Source: CAD feature listing. Evaluate the final solid. Frame: model axes, mm. A direction names the side the tool comes from. Coordinates: 2 decimals unless noted, no trailing zeros. Write each loop counter-clockwise with the first axis right and the second up, starting at its lowest first coordinate (ties: lowest second). Pieces come first, ordered by that corner, then holes. Notation, with made-up numbers: (57.25, 78.25) -> (100.25, 78.25) arc R15 cw to (100.25, 104.25) -> close; hole circle Ø9 at (52, 58.25). An arc over 180 degrees is marked (long way). Write item = value, one per line.
from build123d import *

# Parameters (mm, degrees)
PAD009_DEPTH          = 23
PAD010_DEPTH          = 44
SKETCH024_W           = 43
SKETCH024_H           = 50
POCKET012_DEPTH       = 46
PAD011_DEPTH          = 25
SKETCH026_R           = 1.5
POCKET013_DEPTH       = 44.001
SKETCH027_R           = 3
POCKET014_DEPTH       = 10
POLARPATTERN001_COUNT = 4
POCKET011_DEPTH       = 6
PAD008_DEPTH          = 44
POCKET015_DEPTH       = 64.001
PAD013_DEPTH          = 64
SKETCH032_W           = 40
SKETCH032_H           = 10.43081
POCKET016_DEPTH       = 23.545613
SKETCH033_R           = 1.5
POCKET017_DEPTH       = 83.001
SKETCH034_R           = 4
POCKET018_DEPTH       = 80.001
SKETCH036_R           = 1.5
POCKET019_DEPTH       = 5
SKETCH037_R           = 3
POCKET020_DEPTH       = 10
SKETCH052_W           = 20
SKETCH052_H           = 20
PAD024_DEPTH          = 5
FILLET_R              = 8
FILLET001_R           = 3


with BuildPart() as part:
    # Sketch022 → Pad009 (new body)
    with BuildSketch(Plane.XY):
        Polygon((32, -51), (32, 32), (-32, 32), (-32, -51), (-20, -51), (-20, 20), (20, 20), (20, -51), align=None)
    extrude(amount=-PAD009_DEPTH)

    # Sketch023 (on Face10 of Pad009) → Pad010 (join)
    with BuildSketch(Plane(origin=(0, 0, -23), x_dir=(1, 0, 0), z_dir=(0, 0, -1))):
        with BuildLine():
            Line((-25, 51), (-25, -1))
            Line((-25, -1), (25, -1))
            Line((25, -1), (25, 51))
            Line((25, 51), (11.999997, 51))
            Line((11.999997, 27.99216), (11.999997, 51))
            ThreePointArc((-11.999997, 28.007844), (-0.007842, 16.000003), (11.999997, 27.99216))
            Line((-11.999997, 28.007844), (-11.999997, 51))
            Line((-11.999997, 51), (-25, 51))
        make_face()
    extrude(amount=PAD010_DEPTH)

    # Sketch024 (on Face18 of Pad010) → Pocket012 (cut)
    with BuildSketch(Plane.XZ.offset(51)):
        with Locations((-0.015156, -53)):
            Rectangle(SKETCH024_W, SKETCH024_H)
    extrude(amount=-POCKET012_DEPTH, mode=Mode.SUBTRACT)

    # Sketch025 (on Face14 of Pocket012) → Pad011 (join)
    with BuildSketch(Plane.XZ.offset(51)):
        Polygon((-32, -23), (-25, -23), (-25, -42.561909), align=None)
        Polygon((32, -23), (25, -23), (25, -42.561909), align=None)
    extrude(amount=-PAD011_DEPTH)

    # Sketch026 (on Face11 of Pad011) → Pocket013 (cut, through all)
    with BuildSketch(Plane.XY.offset(-23)):
        with Locations((-15.5, -12.5)):
            Circle(SKETCH026_R)
        with Locations((-15.5, -43.5)):
            Circle(SKETCH026_R)
        with Locations((15.5, -43.5)):
            Circle(SKETCH026_R)
        with Locations((15.5, -12.5)):
            Circle(SKETCH026_R)
    extrude(amount=-POCKET013_DEPTH, mode=Mode.SUBTRACT)

    # Sketch027 (on Face4 of Pocket013) → Pocket014 (cut)
    with BuildSketch(Plane.XY):
        with Locations((-25, 25)):
            Circle(SKETCH027_R)
    pocket014 = extrude(amount=-POCKET014_DEPTH, mode=Mode.SUBTRACT)

    # PolarPattern001: Pocket014 ×4 about axis
    polarpattern001_axis = Axis((0, 0, 0), (0, 0, 1))
    for i in range(1, POLARPATTERN001_COUNT):
        add(pocket014.rotate(polarpattern001_axis, i * 360 / POLARPATTERN001_COUNT), mode=Mode.SUBTRACT)

    # Sketch028 (on Face23 of PolarPattern001) → Pocket011 (cut)
    with BuildSketch(Plane(origin=(0, 1, 0), x_dir=(-1, 0, 0), z_dir=(0, 1, 0))):
        with BuildLine():
            Line((-11.999999, -62.717157), (12.000001, -62.717157))
            Line((12.000001, -62.717157), (12.000001, -49.356773))
            ThreePointArc((12.000001, -49.356773), (1e-06, -37.356773), (-11.999999, -49.356773))
            Line((-11.999999, -49.356773), (-11.999999, -62.717157))
        make_face()
    extrude(amount=-POCKET011_DEPTH, mode=Mode.SUBTRACT)

    # Sketch021 (on Face6 of Pocket011) → Pad008 (join)
    with BuildSketch(Plane(origin=(0, 0, -23), x_dir=(1, 0, 0), z_dir=(0, 0, -1))):
        Polygon((-32, 17), (-25, 17), (-25, 7), (-17, -1), (-17, -15), (-12, -20), (12, -20), (17, -15), (17, -1), (25, 7), (25, 17), (32, 17), (32, -27), (27, -32), (-27, -32), (-32, -27), align=None)
    extrude(amount=PAD008_DEPTH)

    # Sketch029 (on Face52 of Pad008) → Pocket015 (cut, through all)
    with BuildSketch(Plane(origin=(-32, 0, 0), x_dir=(0, -1, 0), z_dir=(-1, 0, 0))):
        with BuildLine():
            Line((7, 0), (-13, 0))
            Line((-13, -62), (-13, 0))
            Line((-13, -62), (0, -62))
            ThreePointArc((0, -62), (4.949747, -59.949747), (7, -55))
            Line((7, -55), (7, 0))
        make_face()
    extrude(amount=-POCKET015_DEPTH, mode=Mode.SUBTRACT)

    # Sketch031 (on Face10 of Pocket015) → Pad013 (join)
    with BuildSketch(Plane(origin=(-32, 0, 0), x_dir=(0, -1, 0), z_dir=(-1, 0, 0))):
        Polygon((51, 0), (51, 23.544613), (32.56919, 0), align=None)
    extrude(amount=-PAD013_DEPTH)

    # Sketch032 (on Face54 of Pad013) → Pocket016 (cut, through all)
    with BuildSketch(Plane(origin=(0, 0, 0), x_dir=(1, 0, 0), z_dir=(0, 0, -1))):
        with Locations((0, 37.784595)):
            Rectangle(SKETCH032_W, SKETCH032_H)
    extrude(amount=-POCKET016_DEPTH, mode=Mode.SUBTRACT)

    # Sketch033 (on Face19 of Pocket016) → Pocket017 (cut, through all)
    with BuildSketch(Plane.XZ.offset(51)):
        with Locations((-24.5, 8)):
            Circle(SKETCH033_R)
        with Locations((24.5, 8)):
            Circle(SKETCH033_R)
    extrude(amount=-POCKET017_DEPTH, mode=Mode.SUBTRACT)

    # Sketch034 (on Face19 of Pocket017) → Pocket018 (cut, through all)
    with BuildSketch(Plane.XZ.offset(48)):
        with Locations((-24.5, 8)):
            Circle(SKETCH034_R)
        with Locations((24.5, 8)):
            Circle(SKETCH034_R)
    extrude(amount=-POCKET018_DEPTH, mode=Mode.SUBTRACT)

    # Sketch036 (on Face6 of Pocket018) → Pocket019 (cut)
    with BuildSketch(Plane.XY.offset(-62)):
        with Locations((24.5, 7)):
            Circle(SKETCH036_R)
        with Locations((-24.5, 7)):
            Circle(SKETCH036_R)
    extrude(amount=-POCKET019_DEPTH, mode=Mode.SUBTRACT)

    # Sketch037 (on Face43 of Pocket019) → Pocket020 (cut)
    with BuildSketch(Plane.XY):
        with Locations((-24.5, 7)):
            Circle(SKETCH037_R)
        with Locations((24.5, 7)):
            Circle(SKETCH037_R)
    extrude(amount=-POCKET020_DEPTH, mode=Mode.SUBTRACT)

    # Sketch052 (on Face17 of Pocket020) → Pad024 (join)
    with BuildSketch(Plane.YZ.offset(32)):
        with Locations((3, -30)):
            Rectangle(SKETCH052_W, SKETCH052_H)
    pad024 = extrude(amount=-PAD024_DEPTH)

    # Mirrored002: Pad024 across YZ
    add(pad024.mirror(Plane.YZ))

    # Fillet
    fillet_edges = [part.edges().sort_by_distance(p)[0] for p in [
        (29.5, -7, -20),
        (29.5, 13, -20),
        (29.5, 13, -40),
        (29.5, -7, -40),
        (-29.5, -7, -20),
        (-29.5, 13, -20),
        (-29.5, -7, -40),
        (-29.5, 13, -40),
    ]]
    fillet(fillet_edges, radius=FILLET_R)

    # Fillet001
    fillet001_edges = [part.edges().sort_by_distance(p)[0] for p in [
        (24.5, 13, -62),
        (-24.5, 13, -62),
    ]]
    fillet(fillet001_edges, radius=FILLET001_R)


solid = part.part
1) Cut plane B-B, the plane z = -52. Output: boundary loops of the cut face in (x, y), and give its area (3 significant figures).
Answer block:
outline = (-32, -17) -> (-25, -17) -> (-25, -51) -> (-21.52, -51) -> (-21.52, -7) -> (-32, -7) -> close; (-32, 13) -> (-17, 13) -> (-17, 15) -> (-12, 20) -> (12, 20) -> (17, 15) -> (17, 13) -> (32, 13) -> (32, 27) -> (27, 32) -> (-27, 32) -> (-32, 27) -> close; (21.48, -51) -> (25, -51) -> (25, -17) -> (32, -17) -> (32, -7) -> (21.48, -7) -> close
area = 1,430 mm2
2) First-contact query: pin 1 Ø1 at (x, y) = (-11, -10) entering from +Z; pin 2 Ø10 at (y, z) = (-35.5, -35) entering from +X; pin 3 Ø6.5 at (x, y) = (-0.5, -46) entering from -Z. Flat tips, straight axial feed; report the tip coordinate or a pass-through.
Answer block:
pin_1 = -23
pin_2 = 29.5
pin_3 = 0
3) Cut plane C-C, the plane y = 25. Output: boundary loops of the cut face in (x, z), and give its area (3 significant figures).
Answer block:
outline = (-32, -67) -> (32, -67) -> (32, 0) -> (28, 0) -> (28, -10) -> (22, -10) -> (22, 0) -> (-22, 0) -> (-22, -10) -> (-28, -10) -> (-28, 0) -> (-32, 0) -> close
area = 4,170 mm2
4) Reachability of faces 4 (the flat face through (24, 5, -62)), 5 (the cylindrical face through (23.633, -43.303, 4.095)), 6 (the flat face through (28, -26, -30)), 7 (the flat face through (-12, -39, -25)), 8 (the cylindrical face through (15.175, -44.964, -25.465)) from +Z, -Z, +X, -X, +Y, -Y: full face, straight path, thin tool, end or side. Return the list, or none.
Answer block:
face_4 = +X, -X
face_5 = +Y
face_6 = -Z, +X
face_7 = -Z, -Y
face_8 = -Z
5) Cut plane A-A, the plane x = 15.5. Output: boundary loops of the cut face in (y, z), and give its area (3 significant figures).
Answer block:
outline = (-51, -28) -> (-45, -28) -> (-45, -23) -> (-51, -23) -> close; (-51, 0) -> (-43, 0) -> (-43, 13.32) -> (-51, 23.54) -> close; (-42, -28) -> (-14, -28) -> (-14, -23) -> (-42, -23) -> close; (-11, -28) -> (-7, -28) -> (-7, -23) -> (-11, -23) -> close; (-5, -67) -> (1, -67) -> (1, -62) -> (0, -62) arc R7 cw to (-5, -59.9) -> close; (16.5, -67) -> (32, -67) -> (32, 0) -> (20, 0) -> (20, -23) -> (16.5, -23) -> close
area = 1,330 mm2
6) Material intervals for probe 1 along X at (y, z) = (-25, -5); probe 2 along Y at (x, z) = (-26, -46.5); probe 3 along Y at (x, z) = (15.5, -24.7), sorted ascending. Write a range as [from, to].
Answer block:
probe_1 = [-32, -28], [-22, -20], [20, 22], [28, 32]
probe_2 = [-17, -7], [13, 32]
probe_3 = [-51, -45], [-42, -14], [-11, -7], [16.5, 32]
7) Pull-direction query (Z, two-part tool) for faces 1 (the flat face through (0, -15, -28)), 2 (the flat face through (20, 17, -11)), 3 (the cylindrical face through (24.6, 12.14, -61.1)); classes: +Z half, -Z half, draft (parallel to the pull), parting line (faces both ways), or undercut.
Answer block:
face_1 = -Z half
face_2 = draft
face_3 = undercut
8) Cut plane D-D, the plane y = 7. Output: boundary loops of the cut face in (x, z), and give its area (3 significant figures).
Answer block:
outline = (-32, -67) -> (-26, -67) -> (-26, -62) -> (-32, -62) -> close; (-32, -40.25) -> (-27, -40.25) -> (-27, -19.75) -> (-32, -19.75) -> close; (-23, -67) -> (-17, -67) -> (-17, -62) -> (-23, -62) -> close; (17, -67) -> (23, -67) -> (23, -62) -> (17, -62) -> close; (26, -67) -> (32, -67) -> (32, -62) -> (26, -62) -> close; (27, -40.25) -> (32, -40.25) -> (32, -19.75) -> (27, -19.75) -> close
area = 325 mm2
